from build123d import *

# Parameters (mm, degrees)
F0_W     = 78.74
F0_H     = 58.42
F1_DEPTH = 5.08
F0_W_2   = 88.9
F0_H_2   = 68.58
F2_DEPTH = 25.4
F3_W     = 58.42
F3_H     = 6.883326
F4_DEPTH = 5.08


with BuildPart() as f1:
    # F0 (on Top) → F1 (new body)
    with BuildSketch(Plane.XY):
        with Locations((44.45, 34.29)):
            Rectangle(F0_W, F0_H)
    extrude(amount=F1_DEPTH)

    # F0 (on Top) → F2 (join)
    with BuildSketch(Plane.XY):
        with Locations((44.45, 34.29)):
            Rectangle(F0_W_2, F0_H_2)
        with Locations((44.45, 34.29)):
            Rectangle(F0_W, F0_H, mode=Mode.SUBTRACT)
    extrude(amount=F2_DEPTH)

    # F3 (on face) → F4 (cut)
    with BuildSketch(Plane.YZ.offset(88.9)):
        with Locations((34.29, 8.521663)):
            Rectangle(F3_W, F3_H)
    extrude(amount=-F4_DEPTH, mode=Mode.SUBTRACT)


solid = f1.part
Geometry check sheet. Reference: the model listing, model coordinates, mm. A direction names the side the tool comes from. Coordinates: 2 decimals unless noted, no trailing zeros. Order: outer loops, then holes, each group sorted by start corner. A loop starts at its lowest first (then second) coordinate and runs counter-clockwise, first axis right, second up. Notation, with made-up numbers: (71.5, 9) -> (130.5, 9) arc R26 cw to (130.5, 31) -> close; hole circle Ø4 at (-10.75, -17). An arc over 180 degrees is marked (long way). Use a Markdown table: item, result. Add a question column.
1. Material ranges on L1, parallel to Y at x = 66, z = 16; L2, parallel to X at y = 35, z = 23; L3, parallel to Z at x = 70.5, y = 23.5, recorded low to high.
2. Set-up check for faces 1 (the face through (0, 34, 13)), 2 (the face through (86, 34, 11.963)), 3 (the face through (5.08, 34, 15)): record each of +Z, -Z, +X, -X, +Y, -Y from which the full face is reachable in a straight line by a thin tool's end or side.
3. Cross-section at B-B (z = 9.5). Enter the section's corners in (x, y), and give its area (3 significant figures).
4. Cross-section at C-C (x = 30.5). Enter the section's corners in (y, z).
5. Mould release check, pull along X, two halves, no side actions. Record for faces 4 (the face through (83.82, 34, 19)), 5 (the face through (44, 35, 0)), 6 (the face through (88.9, 34, 13)), 7 (the face through (46, 63.5, 15)): pulls with the +X half, pulls with the -X half, needs draft (parallel to the pull), parting line crosses it, or undercut.
6. Go/stop test with flat-tipped pins: pin 1 Ø6 at (y, z) = (33.5, 11.5) entering from +X; pin 2 Ø4 at (x, y) = (29.5, 59.5) entering from +Z. Record where each tip stops, or that it passes through.
7. Cross-section at D-D (z = 17.75). Enter the section's corners in (x, y).
8. Cross-section at A-A (y = 15.5). Enter the section's corners in (x, z), and give its area (3 significant figures).
Filled sheet:
| question | item | result |
|---|---|---|
| 1 | L1 | 0 to 5.08, 63.5 to 68.58 |
| 1 | L2 | 0 to 5.08, 83.82 to 88.9 |
| 1 | L3 | 0 to 5.08 |
| 2 | face 1 | +Z, -Z, -X, +Y, -Y |
| 2 | face 2 | +X |
| 2 | face 3 | +Z |
| 3 | outline | (0, 0) -> (88.9, 0) -> (88.9, 5.08) -> (5.08, 5.08) -> (5.08, 63.5) -> (88.9, 63.5) -> (88.9, 68.58) -> (0, 68.58) -> close |
| 3 | area | 1,200 mm2 |
| 4 | outline | (0, 0) -> (68.58, 0) -> (68.58, 25.4) -> (63.5, 25.4) -> (63.5, 5.08) -> (5.08, 5.08) -> (5.08, 25.4) -> (0, 25.4) -> close |
| 5 | face 4 | undercut |
| 5 | face 5 | needs draft |
| 5 | face 6 | pulls with the +X half |
| 5 | face 7 | undercut |
| 6 | pin 1 | x = 88.9 |
| 6 | pin 2 | z = 5.08 |
| 7 | outline | (0, 0) -> (88.9, 0) -> (88.9, 68.58) -> (0, 68.58) -> close; hole (5.08, 5.08) -> (83.82, 5.08) -> (83.82, 63.5) -> (5.08, 63.5) -> close |
| 8 | outline | (0, 0) -> (88.9, 0) -> (88.9, 5.08) -> (5.08, 5.08) -> (5.08, 25.4) -> (0, 25.4) -> close; (83.82, 11.96) -> (88.9, 11.96) -> (88.9, 25.4) -> (83.82, 25.4) -> close |
| 8 | area | 623 mm2 |
